```python
from build123d import *

# Parameters (mm, degrees)
F0_W     = 123
F0_H     = 6
F0_W_2   = 6
F0_H_2   = 63
F1_DEPTH = 3
F2_DEPTH = 35
F3_R     = 1.5
F4_DEPTH = 2


with BuildPart() as f1:
    # F0 (on Top) → F1 (new body)
    with BuildSketch(Plane.XY):
        with Locations((0, 34.5)):
            Rectangle(F0_W, F0_H)
        with Locations((-64.5, 0)):
            Rectangle(F0_W_2, F0_H_2)
        with Locations((-64.5, -34.5)):
            Rectangle(F0_W_2, F0_H)
        with Locations((0, -34.5)):
            Rectangle(F0_W, F0_H)
        with Locations((64.5, 0)):
            Rectangle(F0_W_2, F0_H_2)
        with Locations((64.5, -34.5)):
            Rectangle(F0_W_2, F0_H)
        with Locations((64.5, 34.5)):
            Rectangle(F0_W_2, F0_H)
        with Locations((-64.5, 34.5)):
            Rectangle(F0_W_2, F0_H)
    extrude(amount=F1_DEPTH)

    # F0 (on Top) → F2 (join)
    with BuildSketch(Plane.XY):
        with Locations((-64.5, -34.5)):
            Rectangle(F0_W_2, F0_H)
        with Locations((64.5, -34.5)):
            Rectangle(F0_W_2, F0_H)
        with Locations((64.5, 34.5)):
            Rectangle(F0_W_2, F0_H)
        with Locations((-64.5, 34.5)):
            Rectangle(F0_W_2, F0_H)
    extrude(amount=F2_DEPTH)

    # F3 (on face) → F4 (join)
    with BuildSketch(Plane.XY.offset(35)):
        Polygon((-61.5, 31.5), (-67.5, 31.5), (-60.025126, 24.025126), (-54.025126, 30.025126), (-61.5, 37.5), align=None)
        with Locations((-59.5, 29.5)):
            Circle(F3_R, mode=Mode.SUBTRACT)
    extrude(amount=-F4_DEPTH)


solid = f1.part
```
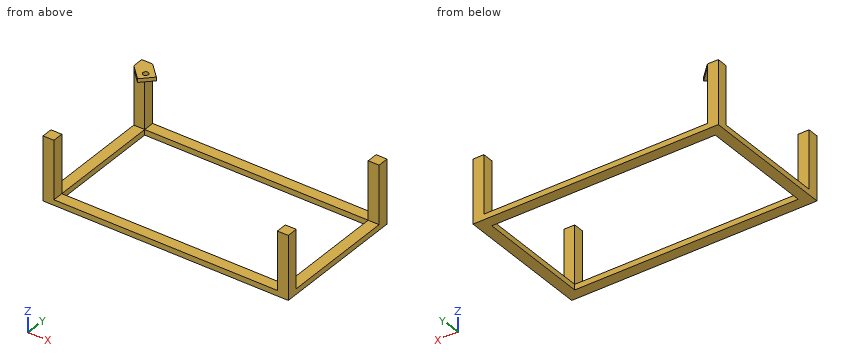
Can you work these out from the model? Positions are in its coordinate system, mm. Round coordinates to 2 decimals unless told otherwise and drop trailing zeros. Loops run counter-clockwise (first coordinate to the right, second up) from the corner with the lowest first, then second, coordinate; pieces in that order, holes last. Notation, with made-up numbers: M -27,88 L 13,88 A18 ccw 13,112 Z; hole C -2.75,39.25 d10. An arc over 180 degrees is marked long. Answer in a Markdown table with one row per item.
1. If we section it at C-C, the plane x = 22.5: Please give me the cut outline in (y, z).
Established:
| item | result |
|---|---|
| outline | M -37.5,0 L -31.5,0 L -31.5,3 L -37.5,3 Z; M 31.5,0 L 37.5,0 L 37.5,3 L 31.5,3 Z |
2. If we section it at B-B, the plane z = 23: Please give me the cut outline in (x, y), plus the area to 3 significant figures.
Established:
| item | result |
|---|---|
| outline | M -67.5,-37.5 L -61.5,-37.5 L -61.5,-31.5 L -67.5,-31.5 Z; M -67.5,31.5 L -61.5,31.5 L -61.5,37.5 L -67.5,37.5 Z; M 61.5,-37.5 L 67.5,-37.5 L 67.5,-31.5 L 61.5,-31.5 Z; M 61.5,31.5 L 67.5,31.5 L 67.5,37.5 L 61.5,37.5 Z |
| area | 144 mm² |
3. If we section it at A-A, the plane y = -23.5: Please give me the cut outline in (x, z), plus the area to 3 significant figures.
Established:
| item | result |
|---|---|
| outline | M -67.5,0 L -61.5,0 L -61.5,3 L -67.5,3 Z; M 61.5,0 L 67.5,0 L 67.5,3 L 61.5,3 Z |
| area | 36.0 mm² |
4. Please list where these lines run through material, in increasing order: line 1 (Y direction, x = -10, z = 2); line 2 (X direction, y = 34, z = 24); line 3 (Y direction, x = -59.5, z = 34.2). Write a range as from..to.
Established:
| item | result |
|---|---|
| line 1 | -37.5..-31.5, 31.5..37.5 |
| line 2 | -67.5..-61.5, 61.5..67.5 |
| line 3 | 24.55..28, 31..35.5 |
5. I'm going to push flat-ended pins straight in: pin 1 Ø6.5 at (x, y) = (64, -2) entering from +Z; pin 2 Ø4 at (x, y) = (-62.5, 31) entering from -Z; pin 3 Ø3 at (x, y) = (-43.5, 29) entering from +Z. Where does each tip first touch, or does it pass through?
Established:
| item | result |
|---|---|
| pin 1 | z = 3 |
| pin 2 | z = 0 |
| pin 3 | through |
